Check sheet for the modelled part. Datum: model origin and axes. Units: mm. Round coordinates to 2 decimals unless told otherwise and drop trailing zeros. Order: outer loops, then holes, each group sorted by start corner. A loop starts at its lowest first (then second) coordinate and runs counter-clockwise, first axis right, second up. Notation, with made-up numbers: M 58.25,86.25 L 102.25,86.25 A17 ccw 102.25,90.25 Z; hole C 2.5,41 d2. An arc over 180 degrees is marked long. One line per item, written item: value. Start each with the question number.
(1) Depth check by flat-ended pin: pin 1 Ø3.5 at (x, z) = (0, 218.4) entering from +Y; pin 2 Ø0.8 at (y, z) = (2, 128.5) entering from +X. Enter the tip coordinate at first touch or a pass-through.
(2) Thickness scan on L1, parallel to X at y = -2.45, z = 43.4; L2, parallel to Y at x = 5, z = 14; L3, parallel to X at y = 2, z = 98.5. Record the ranges inside material, lowest first.
(3) Cross-section at B-B, the plane z = 99. Enter the section's corners in (x, y).
(4) Cross-section at A-A, the plane y = -2.5. Count the separate pieces of the cut face and the enclosed holes in it, and give its area (3 significant figures).
from build123d import *

# Parameters (mm, degrees)
SKETCH1_W           = 11.5
SKETCH1_H           = 7.8
BOSS_EXTRUDE1_DEPTH = 230
SKETCH2_W           = 0.835250229
SKETCH2_H           = 1.6
CUT_EXTRUDE1_DEPTH  = 231.104916288
SKETCH3_R           = 3
CUT_EXTRUDE2_DEPTH  = 4.7
SKETCH4_R           = 1.7
CUT_EXTRUDE3_DEPTH  = 231.119865505


with BuildPart() as part:
    # Sketch1 → Boss-Extrude1 (new body)
    with BuildSketch(Plane.XY):
        Rectangle(SKETCH1_W, SKETCH1_H)
    extrude(amount=BOSS_EXTRUDE1_DEPTH)

    # Sketch2 → Cut-Extrude1 (cut, through all)
    with BuildSketch(Plane.XY.offset(230)):
        with Locations((5.332374886, 1.7)):
            Rectangle(SKETCH2_W, SKETCH2_H)
        with Locations((-5.332374886, 1.7)):
            Rectangle(SKETCH2_W, SKETCH2_H)
    extrude(amount=-CUT_EXTRUDE1_DEPTH, mode=Mode.SUBTRACT)

    # Sketch3 → Cut-Extrude2 (cut)
    with BuildSketch(Plane(origin=(0, 3.9, 0), x_dir=(1, 0, 0), z_dir=(0, 1, 0))):
        with Locations(Location((0, -218.4, 0), (0, 0, 270))):
            Circle(SKETCH3_R)
        with Locations(Location((0, -193.4, 0), (0, 0, 270))):
            Circle(SKETCH3_R)
        with Locations(Location((0, -168.4, 0), (0, 0, 270))):
            Circle(SKETCH3_R)
        with Locations(Location((0, -143.4, 0), (0, 0, 270))):
            Circle(SKETCH3_R)
        with Locations(Location((0, -118.4, 0), (0, 0, 270))):
            Circle(SKETCH3_R)
        with Locations(Location((0, -93.4, 0), (0, 0, 270))):
            Circle(SKETCH3_R)
        with Locations(Location((0, -68.4, 0), (0, 0, 270))):
            Circle(SKETCH3_R)
        with Locations(Location((0, -43.4, 0), (0, 0, 270))):
            Circle(SKETCH3_R)
        with Locations(Location((0, -18.4, 0), (0, 0, 270))):
            Circle(SKETCH3_R)
        with Locations((0, 6.6)):
            Circle(SKETCH3_R)
        with Locations((0, 31.6)):
            Circle(SKETCH3_R)
        with Locations((0, 56.6)):
            Circle(SKETCH3_R)
        with Locations((0, 81.6)):
            Circle(SKETCH3_R)
        with Locations((0, 106.6)):
            Circle(SKETCH3_R)
        with Locations((0, 131.6)):
            Circle(SKETCH3_R)
        with Locations((0, 156.6)):
            Circle(SKETCH3_R)
        with Locations((0, 181.6)):
            Circle(SKETCH3_R)
        with Locations((0, 206.6)):
            Circle(SKETCH3_R)
        with Locations((0, 231.6)):
            Circle(SKETCH3_R)
        with Locations((0, 256.6)):
            Circle(SKETCH3_R)
        with Locations((0, 281.6)):
            Circle(SKETCH3_R)
        with Locations((0, 306.6)):
            Circle(SKETCH3_R)
        with Locations((0, 331.6)):
            Circle(SKETCH3_R)
        with Locations((0, 356.6)):
            Circle(SKETCH3_R)
        with Locations((0, 381.6)):
            Circle(SKETCH3_R)
    extrude(amount=-CUT_EXTRUDE2_DEPTH, mode=Mode.SUBTRACT)

    # Sketch4 → Cut-Extrude3 (cut, through all)
    with BuildSketch(Plane(origin=(0, -0.8, 0), x_dir=(1, 0, 0), z_dir=(0, 1, 0))):
        with Locations(Location((0, -218.4, 0), (0, 0, 270))):
            Circle(SKETCH4_R)
        with Locations(Location((0, -193.4, 0), (0, 0, 270))):
            Circle(SKETCH4_R)
        with Locations(Location((0, -168.4, 0), (0, 0, 270))):
            Circle(SKETCH4_R)
        with Locations(Location((0, -143.4, 0), (0, 0, 270))):
            Circle(SKETCH4_R)
        with Locations(Location((0, -118.4, 0), (0, 0, 270))):
            Circle(SKETCH4_R)
        with Locations(Location((0, -93.4, 0), (0, 0, 270))):
            Circle(SKETCH4_R)
        with Locations(Location((0, -68.4, 0), (0, 0, 270))):
            Circle(SKETCH4_R)
        with Locations(Location((0, -43.4, 0), (0, 0, 270))):
            Circle(SKETCH4_R)
        with Locations(Location((0, -18.4, 0), (0, 0, 270))):
            Circle(SKETCH4_R)
        with Locations((0, 6.6)):
            Circle(SKETCH4_R)
        with Locations((0, 31.6)):
            Circle(SKETCH4_R)
        with Locations((0, 56.6)):
            Circle(SKETCH4_R)
        with Locations((0, 81.6)):
            Circle(SKETCH4_R)
        with Locations((0, 106.6)):
            Circle(SKETCH4_R)
        with Locations((0, 131.6)):
            Circle(SKETCH4_R)
        with Locations((0, 156.6)):
            Circle(SKETCH4_R)
        with Locations((0, 181.6)):
            Circle(SKETCH4_R)
        with Locations((0, 206.6)):
            Circle(SKETCH4_R)
        with Locations((0, 231.6)):
            Circle(SKETCH4_R)
        with Locations((0, 256.6)):
            Circle(SKETCH4_R)
        with Locations((0, 281.6)):
            Circle(SKETCH4_R)
        with Locations((0, 306.6)):
            Circle(SKETCH4_R)
        with Locations((0, 331.6)):
            Circle(SKETCH4_R)
        with Locations((0, 356.6)):
            Circle(SKETCH4_R)
        with Locations((0, 381.6)):
            Circle(SKETCH4_R)
    extrude(amount=-CUT_EXTRUDE3_DEPTH, mode=Mode.SUBTRACT)


solid = part.part
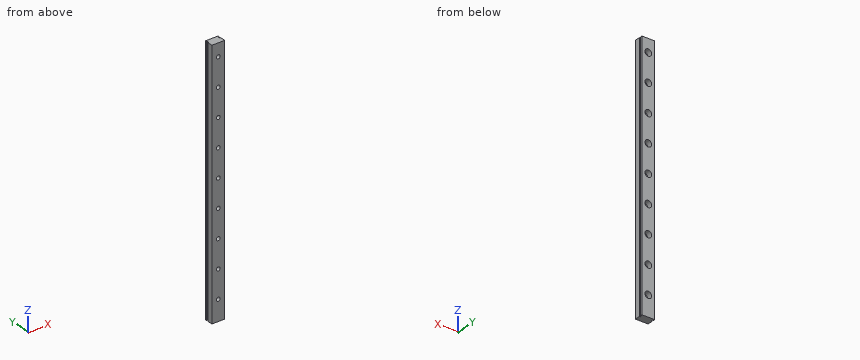
Values found:
1. pin 1: y = -0.8
1. pin 2: x = 4.91
2. L1: -5.75 to -1.7, 1.7 to 5.75
2. L2: -3.9 to 0.9, 2.5 to 3.9
2. L3: -4.91 to 4.91
3. outline: M -5.75,-3.9 L 5.75,-3.9 L 5.75,0.9 L 4.91,0.9 L 4.91,2.5 L 5.75,2.5 L 5.75,3.9 L -5.75,3.9 L -5.75,2.5 L -4.91,2.5 L -4.91,0.9 L -5.75,0.9 Z
4. separate pieces: 1
4. enclosed holes: 9
4. area: 2,560 mm^2
